```python
from build123d import *

# Parameters (mm, degrees)
SKETCH_1_W          = 180
SKETCH_1_H          = 180
EXTRUDE_1_DEPTH     = 2
SKETCH_2_R          = 15
CUT_EXTRUDE_1_DEPTH = 2
CUT_EXTRUDE_2_DEPTH = 3
SKETCH_4_R          = 2.2
CUT_EXTRUDE_3_DEPTH = 160


with BuildPart() as part:
    # ｽｹｯﾁ1 → ﾎﾞｽ - 押し出し1 (new body)
    with BuildSketch(Plane.XY):
        Rectangle(SKETCH_1_W, SKETCH_1_H)
    extrude(amount=EXTRUDE_1_DEPTH)

    # ｽｹｯﾁ2 → ｶｯﾄ - 押し出し1 (cut)
    with BuildSketch(Plane.XY.offset(2)):
        Circle(SKETCH_2_R)
    extrude(amount=-CUT_EXTRUDE_1_DEPTH, mode=Mode.SUBTRACT)

    # ｽｹｯﾁ3 → ｶｯﾄ - 押し出し2 (cut, through all)
    with BuildSketch(Plane(origin=(0, 0, 0), x_dir=(-1, 0, 0), z_dir=(0, 0, -1))):
        with BuildLine():
            ThreePointArc((-52.2, -82.5), (-51.555634919, -84.055634919), (-50, -84.7))
            Line((-50, -84.7), (-50, -82.5))
            Line((-50, -82.5), (-52.2, -82.5))
        make_face()
        with BuildLine():
            Line((-50, -82.5), (-50, -84.7))
            ThreePointArc((-50, -84.7), (-48.444365081, -84.055634919), (-47.8, -82.5))
            ThreePointArc((-47.8, -82.5), (-50, -80.3), (-52.2, -82.5))
            Line((-52.2, -82.5), (-50, -82.5))
        make_face()
        with BuildLine():
            ThreePointArc((52.2, -82.5), (48.444365081, -80.944365081), (50, -84.7))
            Line((50, -84.7), (50, -82.5))
            Line((50, -82.5), (52.2, -82.5))
        make_face()
        with BuildLine():
            Line((50, -82.5), (50, -84.7))
            ThreePointArc((50, -84.7), (51.555634919, -84.055634919), (52.2, -82.5))
            Line((52.2, -82.5), (50, -82.5))
        make_face()
    extrude(amount=-CUT_EXTRUDE_2_DEPTH, mode=Mode.SUBTRACT)

    # ｽｹｯﾁ4 → ｶｯﾄ - 押し出し3 (cut)
    with BuildSketch(Plane(origin=(0, 0, 0), x_dir=(-1, 0, 0), z_dir=(0, 0, -1))):
        with Locations((-82.5, -70)):
            Circle(SKETCH_4_R)
        with Locations((-82.5, 50)):
            Circle(SKETCH_4_R)
        with Locations((82.5, 50)):
            Circle(SKETCH_4_R)
        with Locations((82.5, -70)):
            Circle(SKETCH_4_R)
    extrude(amount=-CUT_EXTRUDE_3_DEPTH, mode=Mode.SUBTRACT)


solid = part.part
```
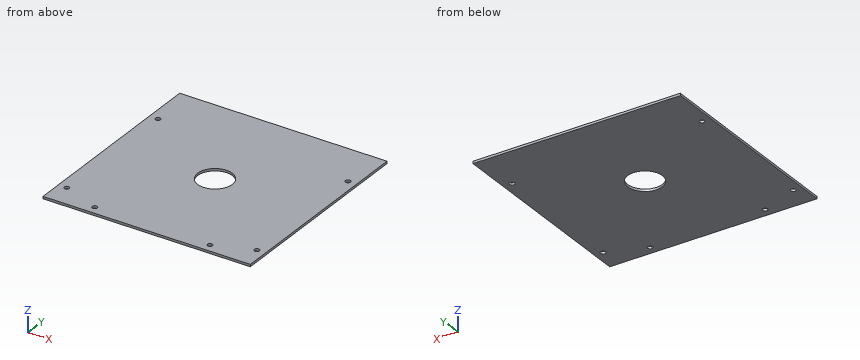
Part model, mm, in its own coordinate system. Round coordinates to 2 decimals unless told otherwise and drop trailing zeros. Loops run counter-clockwise (first coordinate to the right, second up) from the corner with the lowest first, then second, coordinate; pieces in that order, holes last. Notation, with made-up numbers: (-24, 82.25) -> (27, 82.25) arc R13 ccw to (27, 98.25) -> close; hole circle Ø8 at (65.25, -14). An arc over 180 degrees is marked (long way). Use a Markdown table: item, result.
1) Probe line 1 (X direction, y = -82.5, z = 1.05); line 2 (Y direction, x = 82.5, z = 1.4); line 3 (Y direction, x = -50, z = 1.4). List the from-to ranges inside material, lowest first. Write a range as [from, to].
The answers:
| item | result |
|---|---|
| line 1 | x = [-90, -52.2], [-47.8, 47.8], [52.2, 90] |
| line 2 | y = [-90, -72.2], [-67.8, 47.8], [52.2, 90] |
| line 3 | y = [-90, -84.7], [-80.3, 90] |
2) Cut at D-D, the plane y = 3. List the corners of the cut face in (x, z), and give its area (3 significant figures).
The answers:
| item | result |
|---|---|
| outline | (-90, 0) -> (-14.7, 0) -> (-14.7, 2) -> (-90, 2) -> close; (14.7, 0) -> (90, 0) -> (90, 2) -> (14.7, 2) -> close |
| area | 301 mm2 |
3) Cut at B-B, the plane z = 0.3. List the corners of the cut face in (x, y).
The answers:
| item | result |
|---|---|
| outline | (-90, -90) -> (90, -90) -> (90, 90) -> (-90, 90) -> close; hole circle Ø4.4 at (-82.5, -70); hole circle Ø4.4 at (-82.5, 50); hole circle Ø4.4 at (-50, -82.5); hole circle Ø30 at (0, 0); hole circle Ø4.4 at (50, -82.5); hole circle Ø4.4 at (82.5, -70); hole circle Ø4.4 at (82.5, 50) |
4) Cut at C-C, the plane x = -5.5. List the corners of the cut face in (y, z).
The answers:
| item | result |
|---|---|
| outline | (-90, 0) -> (-13.96, 0) -> (-13.96, 2) -> (-90, 2) -> close; (13.96, 0) -> (90, 0) -> (90, 2) -> (13.96, 2) -> close |
5) Cut at A-A, the plane y = 50. List the corners of the cut face in (x, z), and give its area (3 significant figures).
The answers:
| item | result |
|---|---|
| outline | (-90, 0) -> (-84.7, 0) -> (-84.7, 2) -> (-90, 2) -> close; (-80.3, 0) -> (80.3, 0) -> (80.3, 2) -> (-80.3, 2) -> close; (84.7, 0) -> (90, 0) -> (90, 2) -> (84.7, 2) -> close |
| area | 342 mm2 |
